The model under review builds one solid part; all positions refer to its coordinate system, in mm. A direction names the side the tool comes from. Round coordinates to 2 decimals unless told otherwise and drop trailing zeros. Order: outer loops, then holes, each group sorted by start corner. A loop starts at its lowest first (then second) coordinate and runs counter-clockwise, first axis right, second up. Notation, with made-up numbers: (18.25, -34) -> (31.25, -34) arc R22 cw to (31.25, 5) -> close; hole circle Ø4 at (-6, -9). An arc over 180 degrees is marked (long way). Return JSON: item names as keys, results as strings. Group by question number.
from build123d import *

# Parameters (mm, degrees)
SKETCH1_W               = 105
SKETCH1_H               = 105
BOSS_EXTRUDE1_DEPTH     = 12
SKETCH2_R               = 22
SKETCH2_R_2             = 12.5
BOSS_EXTRUDE2_DEPTH     = 96
FILLET1_R               = 5
SKETCH4_R               = 10
CUT_EXTRUDE2_DEPTH      = 2
SKETCH6_R               = 5
CUT_EXTRUDE3_DEPTH      = 11
MIRROR3_COPY_1_SKETCH_R = 10
MIRROR3_COPY_1_DEPTH    = 2
MIRROR3_COPY_2_SKETCH_R = 5
MIRROR3_COPY_2_DEPTH    = 11
BOSS_EXTRUDE5_DEPTH     = 57
SKETCH9_W               = 8
SKETCH9_H               = 16
CUT_EXTRUDE5_DEPTH      = 50
BOSS_EXTRUDE6_DEPTH     = 76
CUT_EXTRUDE6_REACH      = 79.5
SKETCH11_R              = 6
FILLET2_R               = 10
CUT_EXTRUDE7_REACH      = 86.5
SKETCH12_R              = 5


with BuildPart() as part:
    # Sketch1 → Boss-Extrude1 (new body)
    with BuildSketch(Plane.XY):
        Rectangle(SKETCH1_W, SKETCH1_H)
    extrude(amount=BOSS_EXTRUDE1_DEPTH)

    # Sketch2 → Boss-Extrude2 (add)
    with BuildSketch(Plane.XY.offset(12)):
        Circle(SKETCH2_R)
        Circle(SKETCH2_R_2, mode=Mode.SUBTRACT)
    extrude(amount=BOSS_EXTRUDE2_DEPTH)

    # Fillet1
    fillet1_edges = [part.edges().sort_by_distance(p)[0] for p in [
        (-22, 0, 12),
    ]]
    fillet(fillet1_edges, radius=FILLET1_R)

    # Sketch4 → Cut-Extrude2 (cut)
    with BuildSketch(Plane.XY.offset(12)):
        with Locations((-32, 32.5)):
            Circle(SKETCH4_R)
    cut_extrude2 = extrude(amount=-CUT_EXTRUDE2_DEPTH, mode=Mode.SUBTRACT)

    # Sketch6 → Cut-Extrude3 (cut, through all)
    with BuildSketch(Plane.XY.offset(10)):
        with Locations((-32, 32.5)):
            Circle(SKETCH6_R)
    cut_extrude3 = extrude(amount=-CUT_EXTRUDE3_DEPTH, mode=Mode.SUBTRACT)

    # Mirror2: Cut-Extrude2, Cut-Extrude3 across plane
    add(cut_extrude2.mirror(Plane(origin=(0, 0, 0), x_dir=(0, 0, 1), z_dir=(1, 0, 0))), mode=Mode.SUBTRACT)
    add(cut_extrude3.mirror(Plane(origin=(0, 0, 0), x_dir=(0, 0, 1), z_dir=(1, 0, 0))), mode=Mode.SUBTRACT)

    # Mirror3: Cut-Extrude3, Cut-Extrude2 across plane
    add(cut_extrude3.mirror(Plane.ZX), mode=Mode.SUBTRACT)
    add(cut_extrude2.mirror(Plane.ZX), mode=Mode.SUBTRACT)

    # Mirror3 copy 1 sketch → Mirror3 copy 1 (cut)
    with BuildSketch(Plane(origin=(0, 0, 12), x_dir=(-1, 0, 0), z_dir=(0, 0, 1))):
        with Locations((-32, 32.5)):
            Circle(MIRROR3_COPY_1_SKETCH_R)
    extrude(amount=-MIRROR3_COPY_1_DEPTH, mode=Mode.SUBTRACT)

    # Mirror3 copy 2 sketch → Mirror3 copy 2 (cut, through all)
    with BuildSketch(Plane(origin=(0, 0, 10), x_dir=(-1, 0, 0), z_dir=(0, 0, 1))):
        with Locations((-32, 32.5)):
            Circle(MIRROR3_COPY_2_SKETCH_R)
    extrude(amount=-MIRROR3_COPY_2_DEPTH, mode=Mode.SUBTRACT)

    # Sketch8 → Boss-Extrude5 (add)
    with BuildSketch(Plane.XY.offset(108)):
        with BuildLine():
            Line((-32, -22.5), (0, -22))
            ThreePointArc((0, -22), (-9.401774275, -19.889862757), (-17, -13.964240044))
            Line((-17, -13.964240044), (-17, -14))
            Line((-17, -14), (-25, -14))
            Line((-25, -14), (-25, 2))
            Line((-25, 2), (-21.9089023, 2))
            ThreePointArc((-21.9089023, 2), (-21.739374416, 3.37632937), (-21.483471943, 4.739243954))
            Line((-21.483471943, 4.739243954), (-32, 4.739243954))
            Line((-32, 4.739243954), (-32, -22.5))
        make_face()
    extrude(amount=-BOSS_EXTRUDE5_DEPTH)

    # Sketch9 → Cut-Extrude5 (cut)
    with BuildSketch(Plane.XY.offset(108)):
        with Locations((-21, -6)):
            Rectangle(SKETCH9_W, SKETCH9_H)
    extrude(amount=-CUT_EXTRUDE5_DEPTH, mode=Mode.SUBTRACT)

    # Sketch10 → Boss-Extrude6 (add)
    with BuildSketch(Plane.XY.offset(108)):
        with BuildLine():
            Line((-15, 25), (15, 25))
            Line((15, 25), (15, 16.093476939))
            ThreePointArc((15, 16.093476939), (0, 22), (-15, 16.093476939))
            Line((-15, 16.093476939), (-15, 25))
        make_face()
    extrude(amount=-BOSS_EXTRUDE6_DEPTH)

    # Sketch11 → Cut-Extrude6 (cut, up to next)
    with BuildSketch(Plane(origin=(0, 25, 0), x_dir=(1, 0, 0), z_dir=(0, 1, 0)), mode=Mode.PRIVATE) as cut_extrude6_sk1:
        with Locations((0, -88)):
            Circle(SKETCH11_R)
    cut_extrude6_tool1 = extrude(cut_extrude6_sk1.sketch, amount=-CUT_EXTRUDE6_REACH, mode=Mode.PRIVATE) & part.part
    add(cut_extrude6_tool1.solids().sort_by_distance((0, 25, 88))[0], mode=Mode.SUBTRACT)
    # Sketch11 → Cut-Extrude6 (cut, up to next)
    with BuildSketch(Plane(origin=(0, 25, 0), x_dir=(1, 0, 0), z_dir=(0, 1, 0)), mode=Mode.PRIVATE) as cut_extrude6_sk2:
        with Locations((0, -58)):
            Circle(SKETCH11_R)
    cut_extrude6_tool2 = extrude(cut_extrude6_sk2.sketch, amount=-CUT_EXTRUDE6_REACH, mode=Mode.PRIVATE) & part.part
    add(cut_extrude6_tool2.solids().sort_by_distance((0, 25, 58))[0], mode=Mode.SUBTRACT)

    # Fillet2
    fillet2_edges = [part.edges().sort_by_distance(p)[0] for p in [
        (52.5, -52.5, 6),
        (-52.5, -52.5, 6),
        (-52.5, 52.5, 6),
        (52.5, 52.5, 6),
    ]]
    fillet(fillet2_edges, radius=FILLET2_R)

    # Sketch12 → Cut-Extrude7 (cut, up to next)
    with BuildSketch(Plane.ZY.offset(32), mode=Mode.PRIVATE) as cut_extrude7_sk1:
        with Locations((93, -8.880378023)):
            Circle(SKETCH12_R)
    cut_extrude7_tool1 = extrude(cut_extrude7_sk1.sketch, amount=-CUT_EXTRUDE7_REACH, mode=Mode.PRIVATE) & part.part
    add(cut_extrude7_tool1.solids().sort_by_distance((-32, -8.880378, 93))[0], mode=Mode.SUBTRACT)
    # Sketch12 → Cut-Extrude7 (cut, up to next)
    with BuildSketch(Plane.ZY.offset(32), mode=Mode.PRIVATE) as cut_extrude7_sk2:
        with Locations((71, -8.880378023)):
            Circle(SKETCH12_R)
    cut_extrude7_tool2 = extrude(cut_extrude7_sk2.sketch, amount=-CUT_EXTRUDE7_REACH, mode=Mode.PRIVATE) & part.part
    add(cut_extrude7_tool2.solids().sort_by_distance((-32, -8.880378, 71))[0], mode=Mode.SUBTRACT)


solid = part.part
Item 1: Insertion check: pin 1 Ø12 at (x, y) = (-32, 32.5) entering from +Z; pin 2 Ø9.5 at (x, z) = (0, 88) entering from +Y; pin 3 Ø6.5 at (x, z) = (-22.5, 70.5) entering from -Y. Each pin has a flat end and moves straight along its axis. Give the tip position at first contact, or say it passes through.
Item 2: The part is to be moulded in two halves that separate along X. For faces 1 (the face through (-28.549, -10.795, 75.619)), 2 (the face through (49.49, 49.65, 6.08)), 3 (the face through (-25, -6, 80)), 4 (the face through (0, 0, 12)), say which applies: +X half, -X half, draft (parallel to the pull), parting line (faces both ways), or undercut.
Item 3: Consider section C-C on x = 30. State the section outline as (y, z) points.
Item 4: Wall thickness on line 1 along X through (y, z) = (32, 2); line 2 along Y through (x, z) = (-32, 4); line 3 along X through (y, z) = (-32.5, 11.25): over which ranges is each line inside the solid? List them lowest first.
Item 5: Consider section B-B on z = 62. State the section outline as (x, y) points.
Item 6: Consider section D-D on z = 43. State the section outline as (x, y) points, plus the area to 3 significant figures.
Item 7: Consider section A-A on y = 0. State the section outline as (x, z) points, plus the area to 3 significant figures.
Item 8: For faces 5 (the face through (20.32, -8.43, 51.75)), 6 (the face through (0, 23, 32)), 7 (the face through (-2.71, -12.203, 59.328)), 8 (the face through (-15, 20, 71)), 9 (the face through (-36.995, -32.72, 5.07)), list the 3-axis set-ups (+Z, -Z, +X, -X, +Y, -Y) from which the entire face can be reached by the end or side of a thin tool; tool diameter is ignored.
Values:
{
 "1": {"pin 1": "z = 10", "pin 2": "y = -11.56", "pin 3": "y = -22.4"},
 "2": {"face 1": "draft", "face 2": "+X half", "face 3": "undercut", "face 4": "undercut"},
 "3": {"outline": "(-52.5, 0) -> (-37.08, 0) -> (-37.08, 10) -> (-42.3, 10) -> (-42.3, 12) -> (-52.5, 12) -> close; (-27.92, 0) -> (27.92, 0) -> (27.92, 10) -> (22.7, 10) -> (22.7, 12) -> (-22.7, 12) -> (-22.7, 10) -> (-27.92, 10) -> close; (37.08, 0) -> (52.5, 0) -> (52.5, 12) -> (42.3, 12) -> (42.3, 10) -> (37.08, 10) -> close"},
 "4": {"line 1": "-52.5 to -36.97, -27.03 to 27.03, 36.97 to 52.5", "line 2": "-52.5 to -37.5, -27.5 to 27.5, 37.5 to 52.5", "line 3": "-52.5 to -42, -22 to 22, 42 to 52.5"},
 "5": {"outline": "(-32, -22.5) -> (0, -22) arc R22 ccw to (15, 16.09) -> (15, 25) -> (4.47, 25) -> (4.47, 11.67) arc R12.5 cw (long way) to (-4.47, 11.67) -> (-4.47, 25) -> (-15, 25) -> (-15, 16.09) arc R22 ccw to (-21.48, 4.74) -> (-32, 4.74) -> close; hole (-25, -14) -> (-17, -14) -> (-17, 2) -> (-25, 2) -> close"},
 "6": {"outline": "(-15, 16.09) arc R22 ccw (long way) to (15, 16.09) -> (15, 25) -> (-15, 25) -> close; hole circle Ø25 at (0, 0)", "area": "1,180 mm^2"},
 "7": {"outline": "(-52.5, 0) -> (52.5, 0) -> (52.5, 12) -> (27, 12) arc R5 cw to (22, 17) -> (22, 108) -> (12.5, 108) -> (12.5, 12) -> (-12.5, 12) -> (-12.5, 108) -> (-17, 108) -> (-17, 58) -> (-22, 58) -> (-22, 17) arc R5 cw to (-27, 12) -> (-52.5, 12) -> close; (-32, 51) -> (-25, 51) -> (-25, 108) -> (-32, 108) -> close", "area": "3,240 mm^2"},
 "8": {"face 5": "none", "face 6": "+Y", "face 7": "+Z", "face 8": "+Z, -X, +Y", "face 9": "+Z, -Z"}
}
